from build123d import *

# Parameters (mm, degrees)
F3_D     = 19.05
F3_DEPTH = 50.8
F3_TIP   = 5.7231973962


with BuildPart() as f1:
    # F0 (on Front) → F1 (revolve)
    with BuildSketch(Plane.XZ):
        with BuildLine():
            Line((-101.6, 0), (0, 0))
            Line((0, 0), (0, 127))
            Line((0, 127), (-38.1, 127))
            ThreePointArc((-38.1, 127), (-91.5651749151, 89.1056905932), (-76.2, 25.4))
            Line((-76.2, 25.4), (-101.6, 25.4))
            Line((-101.6, 25.4), (-101.6, 0))
        make_face()
    revolve(axis=Axis((0, 0, 63.5), (0, 0, 1)))

    # F3
    with Locations(Plane.XY.offset(127)):
        with Locations((-15.24, 15.24), (15.24, 15.24), (15.24, -15.24), (-15.24, -15.24)):
            Hole(F3_D / 2, depth=F3_DEPTH)
            with Locations((0, 0, -(F3_DEPTH + F3_TIP / 2))):  # 118° drill point
                Cone(0, F3_D / 2, F3_TIP, mode=Mode.SUBTRACT)


solid = f1.part
Build history of the part. All positions in model axes, mm. A direction names the side the tool comes from. Round coordinates to 2 decimals unless told otherwise and drop trailing zeros. Use one line per item in the form item = value.
Q1. Drill centre lines: L1, parallel to X at y = 15.24, z = 93 (3 decimals); L2, parallel to Y at x = 15.24, z = 102 (3 decimals); L3, parallel to Y at x = -15, z = 93. Where is each one in solid material? Low to high.
Conclusion:
L1 = -88.642 to -24.765, -5.715 to 5.715, 24.765 to 88.642
L2 = -83.41 to -24.765, -5.715 to 5.715, 24.765 to 83.41
L3 = -88.68 to -24.76, -5.72 to 5.72, 24.76 to 88.68
Q2. Two-plate mould, pull along X, no slides. Class faces 1 (the cylindrical face through (22.025, 99.184, 12.522)), 2 (the conical face through (-14.35, 16.63, 71.47)), 3 (the flat face through (-1, -1, 127)): released by +X, released by -X, zero draft, split by the parting line, or undercut.
Conclusion:
face_1 = split by the parting line
face_2 = undercut
face_3 = zero draft
Q3. Tool access for faces 4 (the flat face through (1, -1, 0)), 5 (the flat face through (15, -76, 25.4)), 6 (the cylindrical face through (-24.04, -18.89, 101.24)): list every direction of +Z, -Z, +X, -X, +Y, -Y with a clear straight run to the whole face (end or side of a thin tool).
Conclusion:
face_4 = -Z, +X, -X, +Y, -Y
face_5 = none
face_6 = +Z
Q4. Drop flat-ended pins along their axis: P1, Ø6, axis at x = -58.5, y = -30.5, coming from the +Z side; P2, Ø25, axis at x = -15.24, y = -15.24, coming from the +Z side; P3, Ø12, axis at x = 28.5, z = 48, coming from the +Y side; P4, Ø2, axis at x = -29.5, z = 90.5, coming from the -Y side. Give the stop position or say it passes through.
Conclusion:
P1 = 120.85
P2 = 127
P3 = 89.73
P4 = -86.65
Q5. Band-saw the part on A-A, the plane z = 113. State how many separate pieces and enclosed holes the cut face has, then the cut area to 3 significant figures.
Conclusion:
separate_pieces = 1
enclosed_holes = 4
area = 16,400 mm²
